Model file for the job. Use its own axes, mm. Coordinates: 2 decimals unless noted, no trailing zeros. Order: outer loops, then holes, each group sorted by start corner. A loop starts at its lowest first (then second) coordinate and runs counter-clockwise, first axis right, second up. Notation, with made-up numbers: (63, 87.5) -> (76, 87.5) arc R27 cw to (76, 104.5) -> close; hole circle Ø6 at (21.25, 58.5). An arc over 180 degrees is marked (long way). Return JSON: item names as keys, results as strings. Group by question number.
1) Flat gauge pins, fed straight in: pin 1 (2.5 mm diameter, centred on x = 0, z = -90.5, fed in from -Y); pin 2 (1 mm diameter, centred on y = 4, z = 120.5, fed in from +X); pin 3 (5.5 mm diameter, centred on x = 15, z = -24, fed in from +Y); pin 4 (3 mm diameter, centred on x = 14.5, y = -9, fed in from +Z). Where does each tip first touch, or does it go through?
2) Cut at A-A (z = -207.5). Write the cut outline in (x, y), and give its area (3 significant figures).
3) Cut at B-B (y = 11). Write the cut outline in (x, z) (3 decimals), and give its area (3 significant figures).
4) Probe line 1 (Y direction, x = 13, z = 158.5); line 2 (Y direction, x = -5, z = -204); line 3 (X direction, y = 2, z = 198). List the from-to ranges inside material, lowest first.
from build123d import *

# Parameters (mm, degrees)
SKETCH1_R           = 8.001
BOSS_EXTRUDE1_DEPTH = 301.625
SKETCH5_R           = 2.8702
CUT_EXTRUDE1_DEPTH  = 5.826
CHAMFER1_SIZE       = 1.27


with BuildPart() as part:
    # Sketch1 → Boss-Extrude1 (new body, symmetric)
    with BuildSketch(Plane.XY):
        with Locations((0, 9.017)):
            Circle(SKETCH1_R)
        Polygon((-19.8882, -15.494), (-8.89, -15.494), (-4.3688, -10.16), (4.3688, -10.16), (8.89, -15.494), (19.8882, -15.494), (19.8882, -10.668), (9.271, -10.668), (3.81, 1.981383396), (0, 0), (-3.81, 1.981383396), (-9.271, -10.668), (-19.8882, -10.668), align=None)
    extrude(amount=BOSS_EXTRUDE1_DEPTH, both=True)

    # Sketch5 → Cut-Extrude1 (cut, through all)
    with BuildSketch(Plane(origin=(0, -10.668, 0), x_dir=(1, 0, 0), z_dir=(0, 1, 0))):
        with Locations((14.5796, -229.235)):
            Circle(SKETCH5_R)
        with Locations((-14.5796, -229.235)):
            Circle(SKETCH5_R)
        with Locations((-14.5796, -76.835)):
            Circle(SKETCH5_R)
        with Locations((14.5796, -76.835)):
            Circle(SKETCH5_R)
        with Locations((-14.5796, 75.565)):
            Circle(SKETCH5_R)
        with Locations((14.5796, 75.565)):
            Circle(SKETCH5_R)
        with Locations((-14.5796, 227.965)):
            Circle(SKETCH5_R)
        with Locations((14.5796, 227.965)):
            Circle(SKETCH5_R)
    extrude(amount=-CUT_EXTRUDE1_DEPTH, mode=Mode.SUBTRACT)

    # Chamfer1
    chamfer1_edges = [part.edges().sort_by_distance(p)[0] for p in [
        (11.7094, -10.668, -75.565),
        (-17.4498, -10.668, 76.835),
        (11.7094, -10.668, 76.835),
        (-17.4498, -10.668, 229.235),
        (-17.4498, -10.668, -227.965),
        (11.7094, -10.668, -227.965),
        (-17.4498, -10.668, -75.565),
        (11.7094, -10.668, 229.235),
    ]]
    chamfer(chamfer1_edges, length=CHAMFER1_SIZE)


solid = part.part
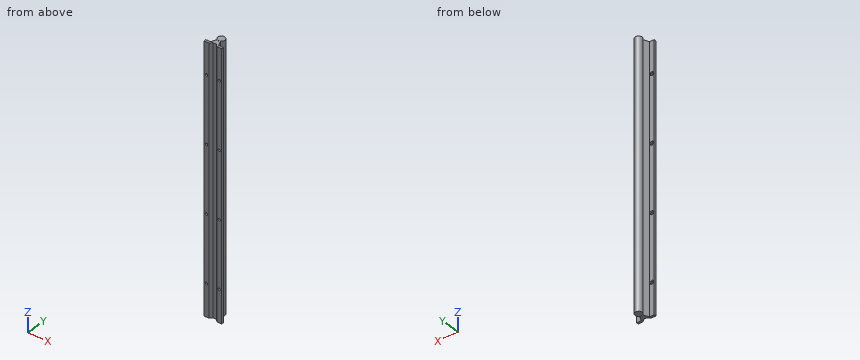
Answers below:
{
 "1": {"pin 1": "stops at y = -10.16", "pin 2": "stops at x = 6.6", "pin 3": "stops at y = -10.67", "pin 4": "passes through"},
 "2": {"outline": "(-19.89, -15.49) -> (-8.89, -15.49) -> (-4.37, -10.16) -> (4.37, -10.16) -> (8.89, -15.49) -> (19.89, -15.49) -> (19.89, -10.67) -> (9.27, -10.67) -> (3.81, 1.98) arc R8 ccw (long way) to (-3.81, 1.98) -> (-9.27, -10.67) -> (-19.89, -10.67) -> close; hole (-3.57, 1.86) -> (0, 0) -> (3.57, 1.86) arc R8 cw to start", "area": "480 mm^2"},
 "3": {"outline": "(-7.751, -301.625) -> (7.751, -301.625) -> (7.751, 301.625) -> (-7.751, 301.625) -> close", "area": "9,350 mm^2"},
 "4": {"line 1": "y = -15.49 to -10.67", "line 2": "y = -10.9 to -0.78, 2.77 to 15.26", "line 3": "x = -3.84 to 3.84"}
}
